from build123d import *

# Parameters (mm, degrees)
F1_DEPTH = 18


with BuildPart() as f1:
    # F0 (on Front) → F1 (new body)
    with BuildSketch(Plane.XZ):
        Polygon((-50, 75), (-50, 0), (50, 0), (50, 75), (75, 75), (75, 225), (50, 225), (50, 275), (75, 275), (75, 425), (50, 425), (50, 575), (75, 575), (75, 725), (50, 725), (50, 775), (75, 775), (75, 925), (50, 925), (50, 1000), (-50, 1000), (-50, 925), (-75, 925), (-75, 775), (-50, 775), (-50, 725), (-75, 725), (-75, 575), (-50, 575), (-50, 425), (-75, 425), (-75, 275), (-50, 275), (-50, 225), (-75, 225), (-75, 75), align=None)
        Polygon((-9, 215), (-9, 225), (9, 225), (9, 215), (40, 215), (40, 160), (9, 160), (9, 140), (40, 140), (40, 85), (9, 85), (9, 75), (-9, 75), (-9, 85), (-40, 85), (-40, 140), (-9, 140), (-9, 160), (-40, 160), (-40, 215), align=None, mode=Mode.SUBTRACT)
        Polygon((-9, 415), (-9, 425), (9, 425), (9, 415), (40, 415), (40, 360), (9, 360), (9, 340), (40, 340), (40, 285), (9, 285), (9, 275), (-9, 275), (-9, 285), (-40, 285), (-40, 340), (-9, 340), (-9, 360), (-40, 360), (-40, 415), align=None, mode=Mode.SUBTRACT)
        Polygon((-9, 715), (-9, 725), (9, 725), (9, 715), (40, 715), (40, 660), (9, 660), (9, 640), (40, 640), (40, 585), (9, 585), (9, 575), (-9, 575), (-9, 585), (-40, 585), (-40, 640), (-9, 640), (-9, 660), (-40, 660), (-40, 715), align=None, mode=Mode.SUBTRACT)
        Polygon((-9, 915), (-9, 925), (9, 925), (9, 915), (40, 915), (40, 860), (9, 860), (9, 840), (40, 840), (40, 785), (9, 785), (9, 775), (-9, 775), (-9, 785), (-40, 785), (-40, 840), (-9, 840), (-9, 860), (-40, 860), (-40, 915), align=None, mode=Mode.SUBTRACT)
    extrude(amount=F1_DEPTH)


solid = f1.part
CAD build for the part. Positions are in the model's coordinates, mm. A direction names the side the tool comes from. Round coordinates to 2 decimals unless told otherwise and drop trailing zeros. Loops run counter-clockwise (first coordinate to the right, second up) from the corner with the lowest first, then second, coordinate; pieces in that order, holes last.
(1) Cut at C-C (z = 502). Give the cut face in (x, y), plus the area to 3 significant figures.
(2) Cut at B-B (y = -2.75). State how many separate pieces and enclosed holes the cut face has, plus the area to 3 significant figures.
(3) Two-plate mould, pull along Z, no slides. Class faces 1 (the flat face through (75, -9, 149)), 2 (the flat face through (62, -9, 75)), 3 (the flat face through (40, -9, 388)): +Z half, -Z half, draft (parallel to the pull), parting line (faces both ways), or undercut.
(4) Drop a flat-ended pin along its axis: pin 1 (9 mm diameter, centred on y = -6.5, z = 471.5, fed in from -X). Give the stop position or say it passes through.
(5) Wall check: line 1 along Z through (x, y) = (-54, -8.75); line 2 along X through (y, z) = (-14.5, 336); line 3 along X through (y, z) = (-14, 653). Give the ranges that are in metal, low to high.
(6) Cut at A-A (z = 897.5). Give the cut face in (x, y), plus the area to 3 significant figures.
(7) Which spindle directions (+Z, -Z, +X, -X, +Y, -Y) get a long thin tool onto all of the face, cutting with end or side? Do faces 4 (the flat face through (-75, -9, 151)), 5 (the flat face through (62, -9, 275)), 6 (the flat face through (-40, -9, 387)). Say none if no direction does.
Findings below:
1. outline: (-50, -18) - (50, -18) - (50, 0) - (-50, 0) - close
1. area: 1,800 mm2
2. separate pieces: 1
2. enclosed holes: 4
2. area: 91,900 mm2
3. face 1: draft
3. face 2: -Z half
3. face 3: undercut
4. pin 1: stops at x = -50
5. line 1: z = 75 to 225, 275 to 425, 575 to 725, 775 to 925
5. line 2: x = -75 to -40, 40 to 75
5. line 3: x = -75 to -9, 9 to 75
6. outline: (-75, -18) - (-40, -18) - (-40, 0) - (-75, 0) - close; (40, -18) - (75, -18) - (75, 0) - (40, 0) - close
6. area: 1,260 mm2
7. face 4: +Z, -Z, -X, +Y, -Y
7. face 5: +X, +Y, -Y
7. face 6: +Y, -Y
